```python
from build123d import *

# Parameters (mm, degrees)
SKETCH1_R             = 12.7
BOSS_EXTRUDE1_DEPTH   = 30.1625
SKETCH4_R             = 15.875
BOSS_EXTRUDE2_DEPTH   = 50.8
CUT_EXTRUDE1_DEPTH    = 11.176
SKETCH3_R             = 6
CUT_EXTRUDE2_DEPTH    = 8
SKETCH5_R             = 3.175
BOSS_EXTRUDE3_DEPTH   = 6.604
F_8_32_TAPPED_HOLE1_D = 3.4544
CUT_EXTRUDE3_START    = -6.35
SKETCH9_R             = 15.875
SKETCH9_R_2           = 6.35
CUT_EXTRUDE3_DEPTH    = 38.1
FILLET1_R             = 3.175
CHAMFER1_SIZE         = 1.27


with BuildPart() as part:
    # Sketch1 → Boss-Extrude1 (new body)
    with BuildSketch(Plane(origin=(0, 0, 0), x_dir=(1, 0, 0), z_dir=(0, 1, 0))):
        Circle(SKETCH1_R)
    extrude(amount=BOSS_EXTRUDE1_DEPTH)

    # Sketch4 → Boss-Extrude2 (add)
    with BuildSketch(Plane(origin=(0, 30.1625, 0), x_dir=(1, 0, 0), z_dir=(0, 1, 0))):
        Circle(SKETCH4_R)
    extrude(amount=BOSS_EXTRUDE2_DEPTH)

    # Sketch2 → Cut-Extrude1 (cut)
    with BuildSketch(Plane.XZ):
        with BuildLine():
            Line((-7, 2.899494937), (-8.776962921, 1.122532015))
            ThreePointArc((-8.776962921, 1.122532015), (-9.241930906, 0), (-8.776962921, -1.122532015))
            Line((-8.776962921, -1.122532015), (-7, -2.899494937))
            Line((-7, -2.899494937), (-7, 2.899494937))
        make_face()
        Polygon((-2.899494937, 7), (-7, 2.899494937), (-7, -2.899494937), (-2.899494937, -7), (2.899494937, -7), (7, -2.899494937), (7, 2.899494937), (2.899494937, 7), align=None)
        with BuildLine():
            Line((-7, 5.4125), (-7, 2.899494937))
            Line((-7, 2.899494937), (-2.899494937, 7))
            Line((-2.899494937, 7), (-5.4125, 7))
            ThreePointArc((-5.4125, 7), (-6.535032015, 6.535032015), (-7, 5.4125))
        make_face()
        with BuildLine():
            Line((-1.122532015, 8.776962921), (-2.899494937, 7))
            Line((-2.899494937, 7), (2.899494937, 7))
            Line((2.899494937, 7), (1.122532015, 8.776962921))
            ThreePointArc((1.122532015, 8.776962921), (0, 9.241930906), (-1.122532015, 8.776962921))
        make_face()
        with BuildLine():
            Line((5.4125, 7), (2.899494937, 7))
            Line((2.899494937, 7), (7, 2.899494937))
            Line((7, 2.899494937), (7, 5.4125))
            ThreePointArc((7, 5.4125), (6.535032015, 6.535032015), (5.4125, 7))
        make_face()
        with BuildLine():
            Line((8.776962921, 1.122532015), (7, 2.899494937))
            Line((7, 2.899494937), (7, -2.899494937))
            Line((7, -2.899494937), (8.776962921, -1.122532015))
            ThreePointArc((8.776962921, -1.122532015), (9.241930906, 0), (8.776962921, 1.122532015))
        make_face()
        with BuildLine():
            Line((7, -2.899494937), (2.899494937, -7))
            Line((2.899494937, -7), (5.4125, -7))
            ThreePointArc((5.4125, -7), (6.535032015, -6.535032015), (7, -5.4125))
            Line((7, -5.4125), (7, -2.899494937))
        make_face()
        with BuildLine():
            Line((2.899494937, -7), (-2.899494937, -7))
            Line((-2.899494937, -7), (-1.122532015, -8.776962921))
            ThreePointArc((-1.122532015, -8.776962921), (0, -9.241930906), (1.122532015, -8.776962921))
            Line((1.122532015, -8.776962921), (2.899494937, -7))
        make_face()
        with BuildLine():
            Line((-2.899494937, -7), (-7, -2.899494937))
            Line((-7, -2.899494937), (-7, -5.4125))
            ThreePointArc((-7, -5.4125), (-6.535032015, -6.535032015), (-5.4125, -7))
            Line((-5.4125, -7), (-2.899494937, -7))
        make_face()
    extrude(amount=-CUT_EXTRUDE1_DEPTH, mode=Mode.SUBTRACT)

    # Sketch3 → Cut-Extrude2 (cut)
    with BuildSketch(Plane.XZ.offset(-11.176)):
        Circle(SKETCH3_R)
    extrude(amount=-CUT_EXTRUDE2_DEPTH, mode=Mode.SUBTRACT)

    # Sketch5 → Boss-Extrude3 (add)
    with BuildSketch(Plane(origin=(0, 80.9625, 0), x_dir=(1, 0, 0), z_dir=(0, 1, 0))):
        Circle(SKETCH5_R)
    extrude(amount=BOSS_EXTRUDE3_DEPTH)

    # #8-32 Tapped Hole1 (through all)
    with Locations(Plane(origin=(0, 87.5665, 0), x_dir=(1, 0, 0), z_dir=(0, 1, 0))):
        with Locations((0, 0)):
            Hole(F_8_32_TAPPED_HOLE1_D / 2)

    # Sketch9 → Cut-Extrude3 (cut)
    with BuildSketch(Plane(origin=(0, 80.9625, 0), x_dir=(1, 0, 0), z_dir=(0, 1, 0)).offset(CUT_EXTRUDE3_START)):
        Circle(SKETCH9_R)
        Circle(SKETCH9_R_2, mode=Mode.SUBTRACT)
    extrude(amount=-CUT_EXTRUDE3_DEPTH, mode=Mode.SUBTRACT)

    # Fillet1
    fillet1_edges = [part.edges().sort_by_distance(p)[0] for p in [
        (-6.35, 36.5125, 0),
        (-6.35, 74.6125, 0),
    ]]
    fillet(fillet1_edges, radius=FILLET1_R)

    # Chamfer1
    chamfer1_edges = [part.edges().sort_by_distance(p)[0] for p in [
        (-15.875, 36.5125, 0),
    ]]
    chamfer(chamfer1_edges, length=CHAMFER1_SIZE)


solid = part.part
```
The listing builds one solid part. Answer for the finished solid, in the listing's coordinates (mm). A direction names the side the tool comes from. Round coordinates to 2 decimals unless told otherwise and drop trailing zeros. Write each loop counter-clockwise with the first axis right and the second up, starting at its lowest first coordinate (ties: lowest second). Pieces come first, ordered by that corner, then holes. Notation, with made-up numbers: (74, 50.5) -> (91, 50.5) arc R17 cw to (91, 60.5) -> close; hole circle Ø7 at (-9, 71.25). An arc over 180 degrees is marked (long way). Answer as a JSON object with one key per item and string values. Group by question number.
Q1. Section A-A (y = 22.5) is taken. Write down the section's boundary in (x, z).
Q2. Straight lines are drawn through the part: line 1 along Y through (x, z) = (-6.5, 7); line 2 along Z through (x, y) = (0, 13); line 3 along Z through (x, y) = (0, 66). For each, find the intervals that lie inside material, in ascending order.
Q3. Each of these flat-tipped pins is pushed along its axis until it touches: pin 1 Ø2 at (y, z) = (5, -4.5) entering from +X; pin 2 Ø1.5 at (y, z) = (55, 5) entering from +X; pin 3 Ø0.8 at (y, z) = (8, -4.5) entering from -X. Where does it stop, or does it pass through?
Q4. Determine the mould class of faces 3 (the face through (0, 80.962, -4)), 4 (the face through (-7.9, 5.5, -2)), 5 (the face through (-3.441, 32.667, 15.497)) for opening direction Z: pulls with the +Z half, pulls with the -Z half, needs draft (parallel to the pull), parting line crosses it, or undercut.
Q5. Section B-B (y = 49.5) is taken. Write down the section's boundary in (x, z).
Q6. Which of the six approach directions +Z, -Z, +X, -X, +Y, -Y give full straight-line access (tool end or side, diameter ignored) to faces 1 (the face through (0.225, 52.893, -1.713)), 2 (the face through (-7, 6, 4))?
Check values:
{
 "1": {"outline": "circle Ø25.4 at (0, 0); hole circle Ø3.45 at (0, 0)"},
 "2": {"line 1": "0 to 36.51, 74.61 to 80.96", "line 2": "-12.7 to -6, 6 to 12.7", "line 3": "-6.35 to -1.73, 1.73 to 6.35"},
 "3": {"pin 1": "x = 12.21", "pin 2": "x = 4.72", "pin 3": "x = -12.02"},
 "4": {"face 3": "needs draft", "face 4": "undercut", "face 5": "parting line crosses it"},
 "5": {"outline": "circle Ø12.7 at (0, 0); hole circle Ø3.45 at (0, 0)"},
 "6": {"face 1": "+Y, -Y", "face 2": "-Y"}
}
